Geometry check sheet. Reference: the model listing, model coordinates, mm. A direction names the side the tool comes from. Round coordinates to 2 decimals unless told otherwise and drop trailing zeros. Use a Markdown table: item, result. Add a question column.
(1) Section check A-A on z = 1. Give the number of separate pieces and of enclosed holes in the cut face, then the cut area to 3 significant figures.
(2) Gauge pin test, flat ends, axial feed: P1, Ø11.5, axis at x = -25.4, y = -50.8, coming from the +Z side; P2, Ø3, axis at x = -18, z = -1.5, coming from the -Y side; P3, Ø3, axis at y = -5, z = -0.5, coming from the +X side; P4, Ø3, axis at x = -22.225, z = 0, coming from the -Y side. Record the tip position at first contact, or that the pin passes through.
(3) Mould release check, pull along X, two halves, no side actions. Record for faces 1 (the face through (31.75, -4, 0)), 2 (the face through (-19.85, -4.7, -0.75)), 3 (the face through (-31.75, -3, 0)), 4 (the face through (-1, -31, 3.175)): released by +X, released by -X, zero draft, split by the parting line, or undercut.
(4) Thickness scan on line 1 along X through (y, z) = (-53, -0.75); line 2 along Y through (x, z) = (25.4, 2) (3 decimals); line 3 along X through (y, z) = (-54.5, -2.25). Record the ranges inside material, lowest first. Write a range as [from, to].
(5) Access from +Z, -Z, +X, -X, +Y, -Y to the whole of each face (thin tool, end or side, straight path). Record for faces 5 (the face through (24.6, -4.7, -0.75)), 6 (the face through (-20, -9.525, 2)), 7 (the face through (19.9, -9.525, 1.5)).
```python
from build123d import *

# Parameters (mm, degrees)
SKETCH1_R                  = 11.43
SKETCH1_R_2                = 6.35
BOSS_EXTRUDE1_DEPTH        = 3.175
FILLET1_R                  = 2.54
F_10_CLEARANCE_HOLE1_D     = 4.9784
F_10_CLEARANCE_HOLE1_DEPTH = 9.525


with BuildPart() as part:
    # Sketch1 → Boss-Extrude1 (new, symmetric)
    # profile 1 of 3: a face of its own
    with BuildSketch(Plane.XY):
        with BuildLine():
            Line((31.75, -9.525), (31.75, 0))
            Line((31.75, 0), (-31.75, 0))
            Line((-31.75, 0), (-31.75, -9.525))
            Line((-31.75, -9.525), (-11.736070368, -9.525))
            add(Edge.make_bspline(
                [(-27.309712652, -39.53066561), (-10.121441585, -36.617924041), (-11.736070368, -9.525)],
                knots=[0, 0, 0, 1, 1, 1], degree=2))
            ThreePointArc((-27.309712652, -39.53066561), (-18.023792154, -42.06865086), (-13.97, -50.8))
            ThreePointArc((-13.97, -50.8), (-14.353544724, -53.736107258), (-15.478438466, -56.47516667))
            add(Edge.make_bspline(
                [(-15.478438466, -56.47516667), (-5.067830393, -38.274910251), (6.38081654, -40.57032704), (15.478438466, -56.47516667)],
                knots=[0, 0, 0, 0, 1, 1, 1, 1], degree=3))
            ThreePointArc((15.478438466, -56.47516667), (16.028422776, -44.256419914), (27.309712652, -39.53066561))
            add(Edge.make_bspline(
                [(27.309712652, -39.53066561), (10.121441585, -36.617924041), (11.736070368, -9.525)],
                knots=[0, 0, 0, 1, 1, 1], degree=2))
            Line((11.736070368, -9.525), (31.75, -9.525))
        make_face()
    # profile 2 of 3: a face of its own
    with BuildSketch(Plane.XY):
        with Locations((-25.4, -50.8)):
            Circle(SKETCH1_R)
        with Locations((-25.4, -50.8)):
            Circle(SKETCH1_R_2, mode=Mode.SUBTRACT)
    # profile 3 of 3: a face of its own
    with BuildSketch(Plane.XY):
        with Locations((25.4, -50.8)):
            Circle(SKETCH1_R)
        with Locations((25.4, -50.8)):
            Circle(SKETCH1_R_2, mode=Mode.SUBTRACT)
    extrude(amount=BOSS_EXTRUDE1_DEPTH, both=True)

    # Fillet1
    fillet1_edges = [part.edges().sort_by_distance(p)[0] for p in [
        (-11.736070368, -9.525, -1.5875),
        (-31.75, -9.525, 0),
        (31.75, -9.525, 0),
        (11.736070368, -9.525, 1.5875),
    ]]
    fillet(fillet1_edges, radius=FILLET1_R)

    # #10 Clearance Hole1
    with Locations(Plane(origin=(0, -9.525, 0), x_dir=(-1, 0, 0), z_dir=(0, -1, 0))):
        with Locations((22.225, 0), (-22.225, 0)):
            Hole(F_10_CLEARANCE_HOLE1_D / 2, depth=F_10_CLEARANCE_HOLE1_DEPTH)


solid = part.part
```
Check sheet entries:
| question | item | result |
|---|---|---|
| 1 | separate pieces | 3 |
| 1 | enclosed holes | 2 |
| 1 | area | 2,210 mm2 |
| 2 | P1 | passes through |
| 2 | P2 | stops at y = -60.59 |
| 2 | P3 | stops at x = 31.75 |
| 2 | P4 | stops at y = -62.11 |
| 3 | face 1 | released by +X |
| 3 | face 2 | undercut |
| 3 | face 3 | released by -X |
| 3 | face 4 | zero draft |
| 4 | line 1 | x = [-36.62, -31.36], [-19.44, -13.31], [13.3, 19.44], [31.36, 36.62] |
| 4 | line 2 | y = [-62.23, -57.15], [-44.45, -39.117], [-9.525, 0] |
| 4 | line 3 | x = [-36.21, -30.56], [-20.24, -14.29], [14.29, 20.24], [30.56, 36.21] |
| 5 | face 5 | +Y |
| 5 | face 6 | +Z, -Z, -X |
| 5 | face 7 | +Z, -Z, +X |
